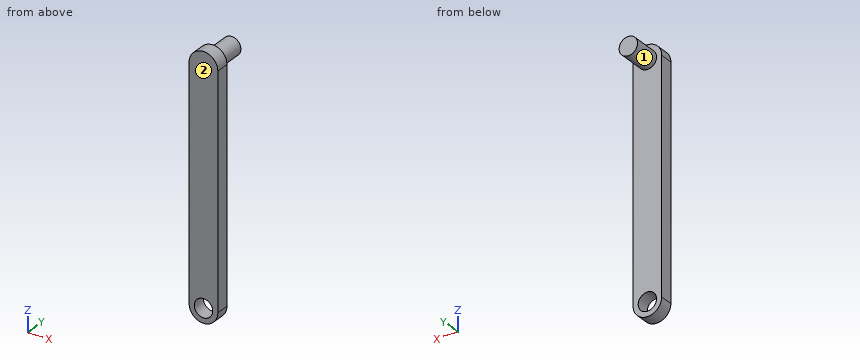
Autodesk Inventor part; units mm, degrees
ref_plane "YZ Plane" through (0, 0, 0) normal (1, 0, 0) x (0, 1, 0)
ref_plane "XZ Plane" through (0, 0, 0) normal (0, 1, 0) x (-1, 0, 0)
ref_plane "XY Plane" through (0, 0, 0) normal (0, 0, 1) x (1, 0, 0)
sketch "Sketch1" plane through (0, 0, 0) normal (0, 1, 0) x (-1, 0, 0)
  line L0 (0, 0) -> (0, -200) construction
  arc A0 (12.5, 0) -> (-12.5, 0) centre (0, 0) ccw
  arc A1 (-12.5, -200) -> (12.5, -200) centre (0, -200) ccw
  line L1 (12.5, -200) -> (12.5, 0)
  line L2 (-12.5, -200) -> (-12.5, 0)
  dimension "d0" = 200
  dimension "d3" = 25
  dimension "d4" = 25
extrude "Extrusion1" add sketch "Sketch1" along normal mid plane 12
sketch "Sketch2" plane through (0, 6, 0) normal (0, 1, 0) x (1, 0, 0)
  circle A0 centre (0, 0) radius 8
  dimension "d7" = 16
extrude "Extrusion2" add sketch "Sketch2" along normal blind 25
sketch "Sketch3" plane through (0, 6, 0) normal (0, 1, 0) x (1, 0, 0)
  circle A0 centre (0, 200) radius 8
  point P0 (0, 0)
  dimension "d10" = 16
extrude "Extrusion3" cut sketch "Sketch3" against normal blind 12
properties part number "manivela"
Design review of the part built by this model. Coordinates are the model's own, in mm. Face numbers are marked on the shaded views. A direction names the side the tool comes from. Coordinates: 2 decimals unless noted, no trailing zeros. Loops run counter-clockwise (first coordinate to the right, second up) from the corner with the lowest first, then second, coordinate; pieces in that order, holes last. Notation, with made-up numbers: (45, -12.75) -> (55, -12.75) arc R25 ccw to (55, 14.25) -> close; hole circle Ø6 at (30, 65.25). An arc over 180 degrees is marked (long way). Answer as a JSON object with one key per item and string values.
Q1. Take a section at C-C on y = 23.5. Give the boundary of the cut face in (x, z), plus the area to 3 significant figures.
Answer block:
{"outline": "circle Ø16 at (0, 0)", "area": "201 mm^2"}
Q2. Clearance check with flat-ended pins moving along their axes: pin 1 Ø5 at (x, y) = (3, 26.5) entering from -Z; pin 2 Ø12 at (x, y) = (4, 25) entering from +Z; pin 3 Ø4 at (x, y) = (9, 23) entering from +Z. State where each tip first meets the part, or that it passes through.
Answer block:
{"pin 1": "stops at z = -7.98", "pin 2": "stops at z = 8", "pin 3": "stops at z = 3.87"}
Q3. Tool access review of the marked faces 1 and 2: name each direction out of +Z, -Z, +X, -X, +Y, -Y from which nothing blocks a thin tool from reaching the whole face with its end or side.
Answer block:
{"face 1": "+Y", "face 2": "+Z, -Z, +X, -X, -Y"}
Q4. Take a section at D-D on z = -108. Give the boundary of the cut face in (x, y), plus the area to 3 significant figures.
Answer block:
{"outline": "(-12.5, -6) -> (12.5, -6) -> (12.5, 6) -> (-12.5, 6) -> close", "area": "300 mm^2"}
Q5. To check wall thickness, follow L1, parallel to Z at x = 0, y = -1; L2, parallel to X at y = 0, z = -200; L3, parallel to Y at x = -0.25, z = -117. State the ranges of each line that lie inside material, in increasing order.
Answer block:
{"L1": "z = -212.5 to -208, -192 to 12.5", "L2": "x = -12.5 to -8, 8 to 12.5", "L3": "y = -6 to 6"}
Q6. Take a section at B-B on y = 3. Give the boundary of the cut face in (x, z).
Answer block:
{"outline": "(-12.5, -200) arc R12.5 ccw to (12.5, -200) -> (12.5, 0) arc R12.5 ccw to (-12.5, 0) -> close; hole circle Ø16 at (0, -200)"}
Q7. Take a section at A-A on x = 0. Give the boundary of the cut face in (y, z).
Answer block:
{"outline": "(-6, -212.5) -> (6, -212.5) -> (6, -208) -> (-6, -208) -> close; (-6, -192) -> (6, -192) -> (6, -8) -> (31, -8) -> (31, 8) -> (6, 8) -> (6, 12.5) -> (-6, 12.5) -> close"}
